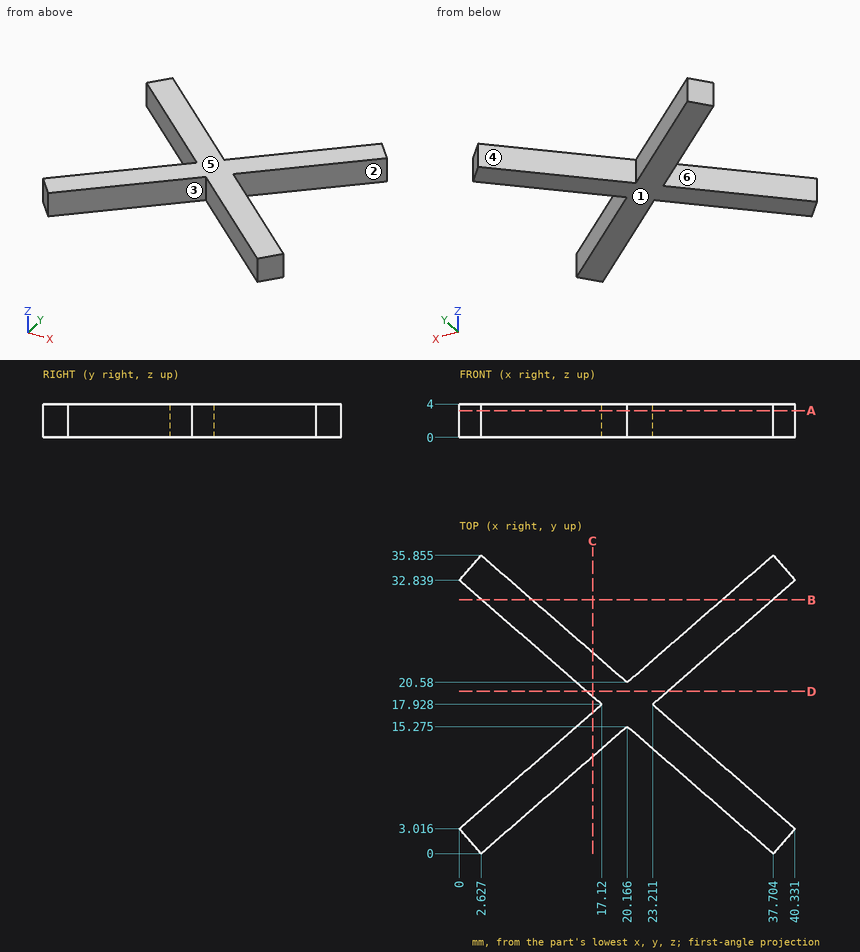
Verification items for this drawing (mm, ordinates from the low corner). A direction names the side the tool comes from. Round coordinates to 2 decimals unless told otherwise and drop trailing zeros. Order: outer loops, then holes, each group sorted by start corner. A loop starts at its lowest first (then second) coordinate and runs counter-clockwise, first axis right, second up.
1) Material ranges on line 1 (X direction, y = 9, z = 2.8); line 2 (Y direction, x = 5, z = 1.15) (1 decimal); line 3 (X direction, y = 27, z = 2.4) (1 decimal), recorded low to high.
Geometry says:
line 1: x = 6.87 to 12.96, 27.37 to 33.46
line 2: y = 2.1 to 7.4, 28.5 to 33.8
line 3: x = 6.7 to 12.8, 27.5 to 33.6
2) Draft check along X on the marked faces 1, 2 and 3. Enter one of: +X half, -X half, draft (parallel to the pull), parting line (faces both ways), or undercut.
Geometry says:
face 1: draft
face 2: +X half
face 3: undercut
3) Cross-section at C-C, the plane x = 16. Record the cut outline in (y, z).
Geometry says:
outline: (11.65, 0) - (16.95, 0) - (16.95, 4) - (11.65, 4) - close; (18.9, 0) - (24.21, 0) - (24.21, 4) - (18.9, 4) - close
4) Cross-section at B-B, the plane y = 30.5. Record the cut outline in (x, z) (1 decimal).
Geometry says:
outline: (2.7, 0) - (8.8, 0) - (8.8, 4) - (2.7, 4) - close; (31.6, 0) - (37.6, 0) - (37.6, 4) - (31.6, 4) - close
5) Tool access check on the marked faces 4, 5 and 6. Record the directions out of +Z, -Z, +X, -X, +Y, -Y that give a thin tool (end or side, any length) a straight path to the whole face; none if there is none.
Geometry says:
face 4: +Z, -Z, +Y
face 5: +Z, +X, -X, +Y, -Y
face 6: +Z, -Z, -X
6) Cross-section at A-A, the plane z = 3.2. Record the cut outline in (x, y) (1 decimal), plus the area to 3 significant figures.
Geometry says:
outline: (0, 3) - (2.6, 0) - (20.2, 15.3) - (37.7, 0) - (40.3, 3) - (23.2, 17.9) - (40.3, 32.8) - (37.7, 35.9) - (20.2, 20.6) - (2.6, 35.9) - (0, 32.8) - (17.1, 17.9) - close
area: 384 mm2
7) Cross-section at D-D, the plane y = 19.5. Record the cut outline in (x, z) (1 decimal), plus the area to 3 significant figures.
Geometry says:
outline: (15.3, 0) - (25, 0) - (25, 4) - (15.3, 4) - close
area: 38.8 mm2
